```python
from build123d import *

# Parameters (mm, degrees)
SKETCH1_W               = 200
SKETCH1_H               = 150
BOSS_EXTRUDE1_DEPTH     = 20
SKETCH2_R               = 7.5
CUT_EXTRUDE1_DEPTH      = 127.589889012
CUT_EXTRUDE2_DEPTH      = 127.589889012
CUT_EXTRUDE2_DEPTH_BACK = 127.589889012
SKETCH3_R               = 1.5
SKETCH4_R               = 0.875
CUT_EXTRUDE3_DEPTH      = 127.589889012


with BuildPart() as part:
    # Sketch1 → Boss-Extrude1 (new body)
    with BuildSketch(Plane(origin=(0, 0, 0), x_dir=(1, 0, 0), z_dir=(0, 1, 0))):
        Rectangle(SKETCH1_W, SKETCH1_H)
    extrude(amount=BOSS_EXTRUDE1_DEPTH)

    # Sketch2 → Cut-Extrude1 (cut, through all)
    with BuildSketch(Plane(origin=(0, 20, 0), x_dir=(1, 0, 0), z_dir=(0, 1, 0))):
        with Locations(Location((-80, 55, 0), (0, 0, 270))):
            Circle(SKETCH2_R)
        with Locations(Location((80, 55, 0), (0, 0, 90))):
            Circle(SKETCH2_R)
        with Locations(Location((-80, -55, 0), (0, 0, 90))):
            Circle(SKETCH2_R)
        with Locations(Location((80, -55, 0), (0, 0, 270))):
            Circle(SKETCH2_R)
    extrude(amount=-CUT_EXTRUDE1_DEPTH, mode=Mode.SUBTRACT)

    # Sketch3 → Cut-Extrude2 (cut, two sides: drawn at the far end of the back side and taken through both)
    with BuildSketch(Plane.XZ.offset(-CUT_EXTRUDE2_DEPTH_BACK)):
        with Locations(Location((-71.5, 8, 0), (0, 0, 270))):
            Circle(SKETCH3_R)
        with Locations(Location((-62.5, 8, 0), (0, 0, 90))):
            Circle(SKETCH3_R)
        with Locations(Location((-62.5, -8, 0), (0, 0, 270))):
            Circle(SKETCH3_R)
        with Locations(Location((-71.5, -8, 0), (0, 0, 90))):
            Circle(SKETCH3_R)
        with Locations(Location((62.5, -8, 0), (0, 0, 90))):
            Circle(SKETCH3_R)
        with Locations(Location((71.5, -8, 0), (0, 0, 270))):
            Circle(SKETCH3_R)
        with Locations(Location((62.5, 8, 0), (0, 0, 270))):
            Circle(SKETCH3_R)
        with Locations(Location((71.5, 8, 0), (0, 0, 90))):
            Circle(SKETCH3_R)
    extrude(amount=CUT_EXTRUDE2_DEPTH + CUT_EXTRUDE2_DEPTH_BACK, mode=Mode.SUBTRACT)

    # Sketch4 → Cut-Extrude3 (cut, through all)
    with BuildSketch(Plane(origin=(0, 20, 0), x_dir=(1, 0, 0), z_dir=(0, 1, 0))):
        with Locations(Location((-18.63, 18.55, 0), (0, 0, 270))):
            Circle(SKETCH4_R)
        with Locations(Location((18.63, 18.55, 0), (0, 0, 90))):
            Circle(SKETCH4_R)
        with Locations(Location((-18.63, -18.55, 0), (0, 0, 90))):
            Circle(SKETCH4_R)
        with Locations(Location((18.63, -18.55, 0), (0, 0, 270))):
            Circle(SKETCH4_R)
    extrude(amount=-CUT_EXTRUDE3_DEPTH, mode=Mode.SUBTRACT)


solid = part.part
```
The listing builds one solid part. Answer for the finished solid, in the listing's coordinates (mm). Coordinates: 2 decimals unless noted, no trailing zeros. Write each loop counter-clockwise with the first axis right and the second up, starting at its lowest first coordinate (ties: lowest second). Pieces come first, ordered by that corner, then holes. Notation, with made-up numbers: M 77,-32.75 L 104,-32.75 A31 cw 104,-7.75 Z; hole C 10,86 d2. An arc over 180 degrees is marked long. Use a Markdown table: item, result. Add a question column.
1. Section A-A (y = 10.75) is taken. Count the separate pieces of the cut face and the enclosed holes in it, plus the area to 3 significant figures.
2. Straight lines are drawn through the part: line 1 along X through (y, z) = (7.25, 55); line 2 along X through (y, z) = (15.5, -8); line 3 along X through (y, z) = (13.25, 18.55) (3 decimals). For each, find the intervals that lie inside material, in ascending order. Write a range as [from, to].
3. Section B-B (x = -84.5) is taken. Give the vertices of the cut face in (y, z).
4. Section C-C (z = -55) is taken. Give the vertices of the cut face in (x, y).
5. For a pull along Z with two mould halves and no side action, classify faces 1 (the flat face through (-1, 0, -1)), 2 (the flat face through (-1, 10, -75)), 3 (the cylindrical face through (86.654, 10.14, -58.461)), 4 (the cylindrical face through (-86.654, 10.14, -51.539)) as +Z half, -Z half, draft (parallel to the pull), parting line (faces both ways), or undercut.
Data:
| question | item | result |
|---|---|---|
| 1 | separate pieces | 1 |
| 1 | enclosed holes | 16 |
| 1 | area | 29,200 mm2 |
| 2 | line 1 | x = [-100, -87.5], [-72.5, 72.5], [87.5, 100] |
| 2 | line 2 | x = [-100, -73], [-70, -64], [-61, 61], [64, 70], [73, 100] |
| 2 | line 3 | x = [-100, -19.505], [-17.755, 17.755], [19.505, 100] |
| 3 | outline | M 0,-75 L 20,-75 L 20,-61 L 0,-61 Z; M 0,-49 L 20,-49 L 20,49 L 0,49 Z; M 0,61 L 20,61 L 20,75 L 0,75 Z |
| 4 | outline | M -100,0 L -87.5,0 L -87.5,20 L -100,20 Z; M -72.5,0 L 72.5,0 L 72.5,20 L -72.5,20 Z; M 87.5,0 L 100,0 L 100,20 L 87.5,20 Z |
| 5 | face 1 | draft |
| 5 | face 2 | -Z half |
| 5 | face 3 | undercut |
| 5 | face 4 | undercut |
